Input: part model. Units: mm. Frame: model coordinates. A direction names the side the tool comes from. Round coordinates to 2 decimals unless told otherwise and drop trailing zeros. Order: outer loops, then holes, each group sorted by start corner. A loop starts at its lowest first (then second) coordinate and runs counter-clockwise, first axis right, second up.
Item 1: Line query: L1, parallel to Y at x = 21, z = -1 (3 decimals); L2, parallel to Z at x = -9, y = -6; L3, parallel to Y at x = 1, z = -12.55 (3 decimals). Output: solid intervals per line, ascending.
Item 2: Cut plane C-C on z = -8.75. Output: boundary loops of the cut face in (x, y) (3 decimals).
Item 3: Cut plane B-B on x = -12. Output: boundary loops of the cut face in (y, z).
Item 4: Mould query, pull axis X, two halves, no side actions, for faces 4 (the flat face through (23.85, 0, 0)), 5 (the cylindrical face through (-22.99, -0.12, -12.95)), 6 (the cylindrical face through (1.33, -4.24, -12.52)). Classes: released by +X, released by -X, zero draft, split by the parting line, or undercut.
Item 5: First-contact query: pin 1 (3.5 mm diameter, centred on x = -12, y = -1.25, fed in from +Z). Flat tip, straight axial feed; report the tip coordinate or a pass-through.
Item 6: Cut plane D-D on y = 4.75. Output: boundary loops of the cut face in (x, z), then the cut area to 3 significant figures.
Item 7: Cut plane A-A on z = -1. Output: boundary loops of the cut face in (x, y) (3 decimals).
Item 8: Reachability of faces 1 (the flat face through (0, -8.75, 12)), 2 (the cylindrical face through (-14.248, -1.151, 11.533)), 3 (the flat face through (0, 0, -11.15)) from +Z, -Z, +X, -X, +Y, -Y: full face, straight path, thin tool, end or side. Return the list, or none.
```python
from build123d import *

# Parameters (mm, degrees)
SKETCH_1_W               = 47.7
SKETCH_1_H               = 27.7
SKETCH_1_W_2             = 30.3
SKETCH_1_H_2             = 20.3
EXTRUDE_1_DEPTH          = 8.75
SKETCH_2_R               = 1.525
CUT_EXTRUDE_1_DEPTH      = 28.7
SKETCH_3_R               = 1.525
CUT_EXTRUDE_2_DEPTH      = 48.7
SKETCH_4_R               = 1.525
CUT_EXTRUDE_3_DEPTH      = 28.7
SKETCH_5_R               = 2.25
CUT_EXTRUDE_4_DEPTH      = 5
SKETCH_7_R               = 1.525
CUT_EXTRUDE_6_DEPTH      = 1
CUT_EXTRUDE_6_DEPTH_BACK = 28.7
CUT_EXTRUDE_7_REACH      = 49.7
SKETCH_8_R               = 1.525
FILLET_2_R               = 3


with BuildPart() as part:
    # 草图1 → 凸台-拉伸1 (new body, symmetric)
    with BuildSketch(Plane(origin=(0, 0, 0), x_dir=(1, 0, 0), z_dir=(0, 1, 0))):
        Rectangle(SKETCH_1_W, SKETCH_1_H)
        with Locations((0, 1)):
            Rectangle(SKETCH_1_W_2, SKETCH_1_H_2, mode=Mode.SUBTRACT)
    extrude(amount=EXTRUDE_1_DEPTH, both=True)

    # 草图2 → 切除-拉伸1 (cut, through all)
    with BuildSketch(Plane(origin=(0, 0, -13.85), x_dir=(-1, 0, 0), z_dir=(0, 0, -1))):
        with Locations((-1, 2.75)):
            Circle(SKETCH_2_R)
    extrude(amount=-CUT_EXTRUDE_1_DEPTH, mode=Mode.SUBTRACT)

    # 草图3 → 切除-拉伸2 (cut, through all)
    with BuildSketch(Plane(origin=(23.85, 0, 0), x_dir=(0, 0, -1), z_dir=(1, 0, 0))):
        with Locations((1, -2.25)):
            Circle(SKETCH_3_R)
    extrude(amount=-CUT_EXTRUDE_2_DEPTH, mode=Mode.SUBTRACT)

    # 草图4 → 切除-拉伸3 (cut, through all)
    with BuildSketch(Plane(origin=(0, 0, -13.85), x_dir=(-1, 0, 0), z_dir=(0, 0, -1))):
        with Locations((19, 2.75)):
            Circle(SKETCH_4_R)
    extrude(amount=-CUT_EXTRUDE_3_DEPTH, mode=Mode.SUBTRACT)

    # 草图5 → 切除-拉伸4 (cut)
    with BuildSketch(Plane.XY.offset(13.85)):
        with Locations((-12, -1.25)):
            Circle(SKETCH_5_R)
        with Locations((12, -1.25)):
            Circle(SKETCH_5_R)
    extrude(amount=-CUT_EXTRUDE_4_DEPTH, mode=Mode.SUBTRACT)

    # 草图7 → 切除-拉伸6 (cut, two sides)
    with BuildSketch(Plane(origin=(0, 0, -13.85), x_dir=(-1, 0, 0), z_dir=(0, 0, -1))) as cut_extrude_6_sk:
        with Locations((-1, -2.75)):
            Circle(SKETCH_7_R)
    extrude(amount=CUT_EXTRUDE_6_DEPTH, mode=Mode.SUBTRACT)
    extrude(cut_extrude_6_sk.sketch, amount=-CUT_EXTRUDE_6_DEPTH_BACK, mode=Mode.SUBTRACT)

    # 草图8 → 切除-拉伸7 (cut, up to next)
    with BuildSketch(Plane(origin=(23.85, 0, 0), x_dir=(0, 0, -1), z_dir=(1, 0, 0)), mode=Mode.PRIVATE) as cut_extrude_7_sk1:
        with Locations((1, 2.25)):
            Circle(SKETCH_8_R)
    cut_extrude_7_tool1 = extrude(cut_extrude_7_sk1.sketch, amount=-CUT_EXTRUDE_7_REACH, mode=Mode.PRIVATE) & part.part
    add(cut_extrude_7_tool1.solids().sort_by_distance((23.85, 2.25, -1))[0], mode=Mode.SUBTRACT)

    # 圆角2
    fillet_2_edges = [part.edges().sort_by_distance(p)[0] for p in [
        (23.85, 0, 13.85),
        (-23.85, 0, 13.85),
        (-23.85, 0, -13.85),
        (23.85, 0, -13.85),
    ]]
    fillet(fillet_2_edges, radius=FILLET_2_R)


solid = part.part
```
From the geometry:
1. L1: y = -8.75 to -3.775, -0.725 to 0.725, 3.775 to 8.75
1. L2: z = -13.85 to -11.15, 9.15 to 13.85
1. L3: y = -8.75 to -4.275, -1.225 to 1.225, 4.275 to 8.75
2. outline: (-23.85, -8.75) - (-15.15, -8.75) - (-15.15, 8.75) - (-23.85, 8.75) - close; (15.15, -8.75) - (23.85, -8.75) - (23.85, 8.75) - (15.15, 8.75) - close; hole circle Ø3.05 at (-19, 2.75)
3. outline: (-8.75, -13.85) - (8.75, -13.85) - (8.75, -11.15) - (-8.75, -11.15) - close; (-8.75, 9.15) - (-3.5, 9.15) - (-3.5, 13.85) - (-8.75, 13.85) - close; (1, 9.15) - (8.75, 9.15) - (8.75, 13.85) - (1, 13.85) - close
4. face 4: released by +X
4. face 5: released by -X
4. face 6: undercut
5. pin 1: stops at z = -11.15
6. outline: (-23.85, -10.85) arc R3 ccw to (-20.85, -13.85) - (20.85, -13.85) arc R3 ccw to (23.85, -10.85) - (23.85, 10.85) arc R3 ccw to (20.85, 13.85) - (-20.85, 13.85) arc R3 ccw to (-23.85, 10.85) - close; hole (-15.15, -11.15) - (15.15, -11.15) - (15.15, 9.15) - (-15.15, 9.15) - close
6. area: 698 mm2
7. outline: (-23.85, -8.75) - (-15.15, -8.75) - (-15.15, -3.775) - (-23.85, -3.775) - close; (-23.85, -0.725) - (-15.15, -0.725) - (-15.15, 8.75) - (-23.85, 8.75) - close; (15.15, -8.75) - (23.85, -8.75) - (23.85, -3.775) - (15.15, -3.775) - close; (15.15, -0.725) - (23.85, -0.725) - (23.85, 0.725) - (15.15, 0.725) - close; (15.15, 3.775) - (23.85, 3.775) - (23.85, 8.75) - (15.15, 8.75) - close; hole circle Ø3.05 at (-19, 2.75)
8. face 1: +Z, -Z, +X, -X, -Y
8. face 2: +Z
8. face 3: +Y, -Y
